Input: part model. Units: mm. Frame: model coordinates. A direction names the side the tool comes from. Coordinates: 2 decimals unless noted, no trailing zeros. Write each loop counter-clockwise with the first axis right and the second up, starting at its lowest first coordinate (ties: lowest second). Pieces come first, ordered by that corner, then holes. Notation, with made-up numbers: (23.5, 47) -> (64.5, 47) arc R17 ccw to (64.5, 55) -> close; hole circle Ø10 at (29, -11). An arc over 180 degrees is marked (long way). Use one line per item in the form item = value. Start each with the question number.
(1) Pull-direction query (X, two-part tool) for faces 5 (the face through (5.72, 189.44, -0.27)), 6 (the face through (6.56, 193.19, 2.92)), 7 (the face through (-6.507, 188.95, 2.868)), 8 (the face through (-3.06, 189.32, -0.32)); classes: released by +X, released by -X, zero draft, split by the parting line, or undercut.
(2) Set-up query: faces 1 (the face through (-6.507, 188.95, -2.868)), 2 (the face through (0, 189, 3.375)), 3 (the face through (6.493, 188.95, -2.882)), 4 (the face through (-7, 189, 0)). Return all of +Z, -Z, +X, -X, +Y, -Y with unobstructed straight access to the full face (end or side cutting, diameter ignored); none if empty.
(3) Cut plane B-B on y = 186. Return the cut outline in (x, z) (3 decimals).
(4) Cut plane A-A on z = 0. Return the cut outline in (x, y), plus the area to 3 significant figures.
(5) First-contact query: pin 1 (4 mm diameter, centred on y = 190, z = -0.5, fed in from -X); pin 2 (3 mm diameter, centred on x = -2.5, y = 188, fed in from +Z) (3 decimals); pin 3 (1.5 mm diameter, centred on y = 188.5, z = 1.5, fed in from +X). Flat tips, straight axial feed; report the tip coordinate or a pass-through.
(6) Ray query, line 1 along X through (y, z) = (191.5, 0); line 2 along Z through (x, y) = (-4.5, 188) (3 decimals); line 3 along Y through (x, z) = (-6.75, 3.25). Return the intervals inside material, ascending.
```python
from build123d import *

# Parameters (mm, degrees)
SKETCH1_W      = 14
SKETCH1_H      = 8.2625
EXTRUDE1_DEPTH = 3.375
SKETCH4_W      = 16
SKETCH4_H      = 8.75
EXTRUDE2_DEPTH = 0.5
SKETCH2_W      = 1.4732
SKETCH2_H      = 14.507045303
SKETCH3_W      = 1.25
SKETCH3_H      = 20
CHAMFER1_SIZE  = 1
FILLET1_R      = 0.25


with BuildPart() as part:
    # Sketch1 → Extrude1 (new body, symmetric)
    with BuildSketch(Plane.XY):
        with Locations((0, 189.13125)):
            Rectangle(SKETCH1_W, SKETCH1_H)
    extrude(amount=EXTRUDE1_DEPTH, both=True)

    # Sketch4 → Extrude2 (add)
    with BuildSketch(Plane(origin=(0, 193.2625, 0), x_dir=(1, 0, 0), z_dir=(0, 1, 0))):
        Rectangle(SKETCH4_W, SKETCH4_H)
    extrude(amount=EXTRUDE2_DEPTH)

    # Sketch2 → Cut-Revolve1 (revolve, cut)
    with BuildSketch(Plane(origin=(9.451328919, 219.930638069, 0), x_dir=(1, 0, 0), z_dir=(0, 0, -1)), mode=Mode.PRIVATE) as cut_revolve1_sk:
        with Locations((-13.214728919, 31.182818604)):
            Rectangle(SKETCH2_W, SKETCH2_H)
    revolve(cut_revolve1_sk.sketch.rotate(Axis((-4.5, 202.803113019, 0), (0, -1, 0)), 90), axis=Axis((-4.5, 202.803113019, 0), (0, -1, 0)), mode=Mode.SUBTRACT)  # turned: the seam where the file's is

    # Sketch3 → Cut-Revolve2 (revolve, cut)
    with BuildSketch(Plane.XY, mode=Mode.PRIVATE) as cut_revolve2_sk:
        with Locations((5.125, 186.074655067)):
            Rectangle(SKETCH3_W, SKETCH3_H)
    revolve(cut_revolve2_sk.sketch.rotate(Axis((4.5, 219.496854939, 0), (0, -1, 0)), 90), axis=Axis((4.5, 219.496854939, 0), (0, -1, 0)), mode=Mode.SUBTRACT)  # turned: the seam where the file's is

    # Chamfer1
    chamfer1_edges = [part.edges().sort_by_distance(p)[0] for p in [
        (7, 189.13125, 3.375),
        (-7, 189.13125, 3.375),
        (7, 189.13125, -3.375),
        (-7, 189.13125, -3.375),
    ]]
    chamfer(chamfer1_edges, length=CHAMFER1_SIZE)

    # Fillet1
    fillet1_edges = [part.edges().sort_by_distance(p)[0] for p in [
        (-7, 193.2625, 0),
        (0, 193.2625, -3.375),
        (7, 193.2625, 0),
        (0, 193.2625, 3.375),
        (-6.5, 193.2625, -2.875),
        (6.5, 193.2625, -2.875),
        (6.5, 193.2625, 2.875),
        (-6.5, 193.2625, 2.875),
    ]]
    fillet(fillet1_edges, radius=FILLET1_R)


solid = part.part
```
Values:
q1.face_5 = undercut
q1.face_6 = released by +X
q1.face_7 = released by -X
q1.face_8 = undercut
q2.face_1 = -Z, -X, -Y
q2.face_2 = +Z, +X, -X, -Y
q2.face_3 = -Z, +X, -Y
q2.face_4 = +Z, -Z, -X, -Y
q3.outline = (-7, -2.375) -> (-6, -3.375) -> (6, -3.375) -> (7, -2.375) -> (7, 2.375) -> (6, 3.375) -> (-6, 3.375) -> (-7, 2.375) -> close; hole circle Ø2.946 at (-4.5, 0); hole circle Ø2.5 at (4.5, 0)
q4.outline = (-8, 193.26) -> (-7.25, 193.26) arc R0.25 cw to (-7, 193.01) -> (-7, 185) -> (-5.97, 185) -> (-5.97, 193.76) -> (-8, 193.76) -> close; (-3.03, 185) -> (3.25, 185) -> (3.25, 193.76) -> (-3.03, 193.76) -> close; (5.75, 185) -> (7, 185) -> (7, 193.01) arc R0.25 cw to (7.25, 193.26) -> (8, 193.26) -> (8, 193.76) -> (5.75, 193.76) -> close
q4.area = 76.0 mm2
q5.pin_1 = -7
q5.pin_2 = 3.375
q5.pin_3 = 7
q6.line_1 = -7 to -5.97, -3.03 to 3.25, 5.75 to 7
q6.line_2 = -3.375 to -1.473, 1.473 to 3.375
q6.line_3 = 193.26 to 193.76
